```python
from build123d import *

# Parameters (mm, degrees)
EXTRUDE_1_DEPTH     = 900
SKETCH_3_OUTSIDE_W  = 2773.258
SKETCH_3_OUTSIDE_H  = 2373.258
CUT_EXTRUDE_3_DEPTH = 1431.244734302


with BuildPart() as part:
    # Эскиз1 → Бобышка-Вытянуть1 (new, symmetric)
    with BuildSketch(Plane.XY):
        with BuildLine():
            Line((-1100, -120), (-1100, 40))
            Line((-1100, 40), (-627.375485654, 40))
            ThreePointArc((-627.375485654, 40), (-589.802028189, 43.561115626), (-553.566604989, 54.117647059))
            ThreePointArc((-553.566604989, 54.117647059), (0, 160), (553.566604989, 54.117647059))
            ThreePointArc((553.566604989, 54.117647059), (589.802028189, 43.561115626), (627.375485654, 40))
            Line((627.375485654, 40), (1100, 40))
            Line((1100, 40), (1100, -120))
            Line((1100, -120), (595.98657703, -120))
            ThreePointArc((595.98657703, -120), (556.509475332, -116.065189265), (518.58572287, -104.415584416))
            ThreePointArc((518.58572287, -104.415584416), (0, 0), (-518.58572287, -104.415584416))
            ThreePointArc((-518.58572287, -104.415584416), (-556.509475332, -116.065189265), (-595.98657703, -120))
            Line((-595.98657703, -120), (-1100, -120))
        make_face()
    extrude(amount=EXTRUDE_1_DEPTH, both=True)

    # Эскиз3 outside → Вырез-Вытянуть3 (cut, through all)
    with BuildSketch(Plane(origin=(0, 40, 0), x_dir=(1, 0, 0), z_dir=(0, 1, 0))):
        Rectangle(SKETCH_3_OUTSIDE_W, SKETCH_3_OUTSIDE_H)
        with BuildLine():
            Line((700, 900), (-700, 900))
            ThreePointArc((-700, 900), (-982.842712475, 782.842712475), (-1100, 500))
            Line((-1100, 500), (-1100, -500))
            ThreePointArc((-1100, -500), (-982.842712475, -782.842712475), (-700, -900))
            Line((-700, -900), (700, -900))
            ThreePointArc((700, -900), (982.842712475, -782.842712475), (1100, -500))
            Line((1100, -500), (1100, 500))
            ThreePointArc((1100, 500), (982.842712475, 782.842712475), (700, 900))
        make_face(mode=Mode.SUBTRACT)
    extrude(amount=-CUT_EXTRUDE_3_DEPTH, mode=Mode.SUBTRACT)


solid = part.part
```
Geometry check sheet. Reference: the model listing, model coordinates, mm. A direction names the side the tool comes from. Give positions to 0.01 mm unless a question says otherwise; leave off trailing zeros. Order: outer loops, then holes, each group sorted by start corner. A loop starts at its lowest first (then second) coordinate and runs counter-clockwise, first axis right, second up.
1. Thickness scan on L1, parallel to X at y = -97, z = -339; L2, parallel to Y at x = -886.5, z = -450.5; L3, parallel to Y at x = -26, z = 277. Record the ranges inside material, lowest first.
2. Gauge pin test, flat ends, axial feed: pin 1 Ø5 at (x, z) = (-60, 345.5) entering from -Y; pin 2 Ø12 at (x, z) = (-576, 40) entering from -Y. Record the tip position at first contact, or that the pin passes through.
3. Section check D-D, the plane z = -668.5. Enter the section's corners in (x, y), and give its area (3 significant figures).
4. Access from +Z, -Z, +X, -X, +Y, -Y to the whole of each face (thin tool, end or side, straight path). Record for faces 1 (the face through (10, 22, 900)), 2 (the face through (557.055, -116.174, 12.6)), 3 (the face through (860, 40, 13)).
5. Section check B-B, the plane z = -66. Enter the section's corners in (x, y), and give its area (3 significant figures).
6. Section check C-C, the plane x = 434. Enter the section's corners in (y, z), and give its area (3 significant figures).
7. Release check for a two-part mould opening along X. For faces 4 (the face through (589.28, 43.66, 12.6)), 5 (the face through (-867, 40, 13)), 6 (the face through (-555.964, -115.955, 12.6)) record: pulls with the +X half, pulls with the -X half, needs draft (parallel to the pull), parting line crosses it, or undercut.
8. Section check A-A, the plane y = -51.5. Enter the section's corners in (x, z).
Values follow:
1. L1: x = -1100 to -500.55, 500.55 to 1100
1. L2: y = -120 to 40
1. L3: y = -0.25 to 159.77
2. pin 1: stops at y = -1.46
2. pin 2: stops at y = -119.51
3. outline: (-1062.78, -120) - (-595.99, -120) arc R200 ccw to (-518.59, -104.42) arc R1340 cw to (518.59, -104.42) arc R200 ccw to (595.99, -120) - (1062.78, -120) - (1062.78, 40) - (627.38, 40) arc R200 cw to (553.57, 54.12) arc R1500 ccw to (-553.57, 54.12) arc R200 cw to (-627.38, 40) - (-1062.78, 40) - close
3. area: 345,000 mm2
4. face 1: +Z, +X, -X, +Y, -Y
4. face 2: +Z, -Z, -Y
4. face 3: +Z, -Z, +X, +Y
5. outline: (-1100, -120) - (-595.99, -120) arc R200 ccw to (-518.59, -104.42) arc R1340 cw to (518.59, -104.42) arc R200 ccw to (595.99, -120) - (1100, -120) - (1100, 40) - (627.38, 40) arc R200 cw to (553.57, 54.12) arc R1500 ccw to (-553.57, 54.12) arc R200 cw to (-627.38, 40) - (-1100, 40) - close
5. area: 357,000 mm2
6. outline: (-72.23, -900) - (95.84, -900) - (95.84, 900) - (-72.23, 900) - close
6. area: 303,000 mm2
7. face 4: pulls with the +X half
7. face 5: needs draft
7. face 6: undercut
8. outline: (-1100, -500) arc R400 ccw to (-700, -900) - (-367.92, -900) - (-367.92, 900) - (-700, 900) arc R400 ccw to (-1100, 500) - close; (367.92, -900) - (700, -900) arc R400 ccw to (1100, -500) - (1100, 500) arc R400 ccw to (700, 900) - (367.92, 900) - close
